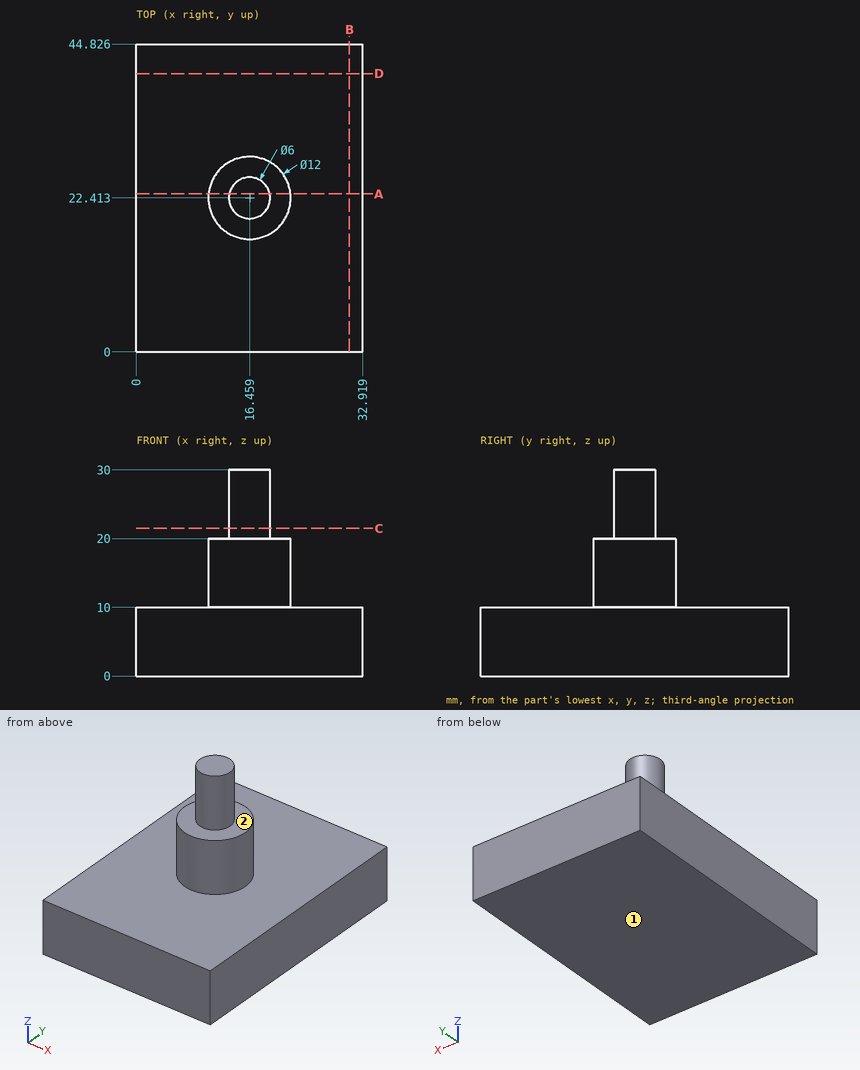
Geometry: see drawing. Coordinates: mm, zero at the bounding-box minimum. A direction names the side the tool comes from. Coordinates: 2 decimals unless noted, no trailing zeros. Order: outer loops, then holes, each group sorted by start corner. A loop starts at its lowest first (then second) coordinate and runs counter-clockwise, first axis right, second up. Notation, with made-up numbers: M -38,74 L 16,74 A11 ccw 16,85 Z; hole C -15,2 d7. An arc over 180 degrees is marked long. Answer as CSV lines item,"result".
1. Section C-C (z = 21.5). Return the cut outline in (x, y), then the cut area to 3 significant figures.
Reported:
outline,"C 16.46,22.41 d6"
area,"28.3 mm2"
2. Section B-B (x = 31). Return the cut outline in (y, z).
Reported:
outline,"M 0,0 L 44.83,0 L 44.83,10 L 0,10 Z"
3. First-contact query: P1, Ø5, axis at x = 27, y = 40, coming from the +Z side; P2, Ø1, axis at x = 26, z = 11, coming from the -Y side. Flat tips, straight axial feed; report the tip coordinate or a pass-through.
Reported:
P1,"z = 10"
P2,"through"
4. Material intervals for line 1 (Z direction, x = 28, y = 4); line 2 (Y direction, x = 14, z = 21) (1 decimal); line 3 (X direction, y = 25, z = 19.5) (1 decimal), sorted ascending. Write a range as from..to.
Reported:
line 1,"0..10"
line 2,"20.7..24.1"
line 3,"11..21.9"
5. Access query for the marked faces 1 and 2. Directions: +Z, -Z, +X, -X, +Y, -Y. A direction counts if a zero-diameter tool reaches every point of the face in a straight line with its end or side. Return the directions, or none.
Reported:
face 1,"-Z, +X, -X, +Y, -Y"
face 2,"+Z"
6. Section D-D (y = 40.5). Return the cut outline in (x, z), then the cut area to 3 significant figures.
Reported:
outline,"M 0,0 L 32.92,0 L 32.92,10 L 0,10 Z"
area,"329 mm2"
7. Section A-A (y = 23). Return the cut outline in (x, z).
Reported:
outline,"M 0,0 L 32.92,0 L 32.92,10 L 22.43,10 L 22.43,20 L 19.4,20 L 19.4,30 L 13.52,30 L 13.52,20 L 10.49,20 L 10.49,10 L 0,10 Z"
